from build123d import *

# Parameters (mm, degrees)
SKETCH1_W                = 74.7
SKETCH1_H                = 52.5
BOSS_EXTRUDE1_DEPTH      = 83
SKETCH4_W                = 42.5
SKETCH4_H                = 42.5
CUT_EXTRUDE1_DEPTH       = 24
SKETCH7_R                = 8.6
CUT_EXTRUDE6_DEPTH       = 130
CUT_EXTRUDE16_DEPTH      = 115.708990493
CUT_EXTRUDE16_DEPTH_BACK = 4.99
SKETCH13_W               = 45.5
SKETCH13_H               = 61
SKETCH15_W               = 6.385819608
SKETCH15_H               = 61
CUT_EXTRUDE17_DEPTH      = 1
SKETCH18_W               = 42.5
SKETCH18_H               = 42.5
BOSS_EXTRUDE2_DEPTH      = 31
SKETCH19_W               = 52.25
SKETCH19_H               = 52.5
BOSS_EXTRUDE3_DEPTH      = 50
SKETCH20_W               = 42.5
SKETCH20_H               = 42.5
CUT_EXTRUDE19_DEPTH      = 23.5
SKETCH21_W               = 52.5
SKETCH21_H               = 5
BOSS_EXTRUDE4_DEPTH      = 30
FILLET1_R                = 5
SKETCH22_R               = 15
CUT_EXTRUDE20_DEPTH      = 120
CUT_EXTRUDE21_DEPTH      = 3
SKETCH24_R               = 20
SKETCH24_R_2             = 15
BOSS_EXTRUDE5_DEPTH      = 82
CUT_EXTRUDE22_START      = -82
CUT_EXTRUDE22_DEPTH      = 82


with BuildPart() as part:
    # Sketch1 → Boss-Extrude1 (new body)
    with BuildSketch(Plane(origin=(0, 0, 0), x_dir=(1, 0, 0), z_dir=(0, 1, 0))):
        Rectangle(SKETCH1_W, SKETCH1_H)
    extrude(amount=BOSS_EXTRUDE1_DEPTH)

    # Sketch4 → Cut-Extrude1 (cut)
    with BuildSketch(Plane.XZ):
        with Locations((11.1, 0)):
            Rectangle(SKETCH4_W, SKETCH4_H)
    extrude(amount=-CUT_EXTRUDE1_DEPTH, mode=Mode.SUBTRACT)

    # Sketch7 → Cut-Extrude6 (cut)
    with BuildSketch(Plane.XZ):
        with Locations(Location((-23.75, 0, 0), (0, 0, 270))):
            Circle(SKETCH7_R)
    extrude(amount=-CUT_EXTRUDE6_DEPTH, mode=Mode.SUBTRACT)

    # Sketch13 → Cut-Extrude16 (cut, two sides: drawn at the far end of the back side and taken through both)
    with BuildSketch(Plane.ZY.offset(37.35).offset(-CUT_EXTRUDE16_DEPTH_BACK)):
        with Locations((0, 41.5)):
            Rectangle(SKETCH13_W, SKETCH13_H)
    extrude(amount=CUT_EXTRUDE16_DEPTH + CUT_EXTRUDE16_DEPTH_BACK, mode=Mode.SUBTRACT)

    # Sketch15 → Cut-Extrude17 (cut)
    with BuildSketch(Plane.ZY.offset(32.36)):
        with Locations((0, 41.5)):
            Rectangle(SKETCH15_W, SKETCH15_H)
    extrude(amount=-CUT_EXTRUDE17_DEPTH, mode=Mode.SUBTRACT)

    # Sketch18 → Boss-Extrude2 (add)
    with BuildSketch(Plane.XZ):
        with Locations((11.1, 0)):
            Rectangle(SKETCH18_W, SKETCH18_H)
    extrude(amount=-BOSS_EXTRUDE2_DEPTH)

    # Sketch19 → Boss-Extrude3 (add)
    with BuildSketch(Plane.XZ):
        with Locations((11.225, 0)):
            Rectangle(SKETCH19_W, SKETCH19_H)
    extrude(amount=BOSS_EXTRUDE3_DEPTH)

    # Sketch20 → Cut-Extrude19 (cut)
    with BuildSketch(Plane.XZ.offset(50)):
        with Locations((11.1, 0)):
            Rectangle(SKETCH20_W, SKETCH20_H)
    extrude(amount=-CUT_EXTRUDE19_DEPTH, mode=Mode.SUBTRACT)

    # Sketch21 → Boss-Extrude4 (add)
    with BuildSketch(Plane(origin=(37.35, 0, 0), x_dir=(0, 0, -1), z_dir=(1, 0, 0))):
        with Locations((0, -47.5)):
            Rectangle(SKETCH21_W, SKETCH21_H)
    extrude(amount=BOSS_EXTRUDE4_DEPTH)

    # Fillet1
    fillet1_edges = [part.edges().sort_by_distance(p)[0] for p in [
        (37.35, -45, 0),
    ]]
    fillet(fillet1_edges, radius=FILLET1_R)

    # Sketch22 → Cut-Extrude20 (cut)
    with BuildSketch(Plane.XZ.offset(26.5)):
        with Locations(Location((11.1, 0, 0), (0, 0, 270))):
            Circle(SKETCH22_R)
    extrude(amount=-CUT_EXTRUDE20_DEPTH, mode=Mode.SUBTRACT)

    # Sketch23 → Cut-Extrude21 (cut)
    with BuildSketch(Plane(origin=(0, 83, 0), x_dir=(1, 0, 0), z_dir=(0, 1, 0))):
        Polygon((-16.75, 16), (-12.788538026, -0.140014893), (-16.75, -16), (-30.75, -16), (-34.596459266, 0.235543482), (-30.75, 16), align=None)
    extrude(amount=-CUT_EXTRUDE21_DEPTH, mode=Mode.SUBTRACT)

    # Sketch24 → Boss-Extrude5 (add)
    with BuildSketch(Plane(origin=(0, 83, 0), x_dir=(1, 0, 0), z_dir=(0, 1, 0))):
        with Locations(Location((11.1, 0, 0), (0, 0, 270))):
            Circle(SKETCH24_R)
        with Locations(Location((11.1, 0, 0), (0, 0, 90))):
            Circle(SKETCH24_R_2, mode=Mode.SUBTRACT)
    extrude(amount=BOSS_EXTRUDE5_DEPTH)

    # Sketch27 → Cut-Extrude22 (cut)
    with BuildSketch(Plane(origin=(0, 165, 0), x_dir=(1, 0, 0), z_dir=(0, 1, 0)).offset(CUT_EXTRUDE22_START)):
        with BuildLine():
            Line((-5.423226258, 11.268673126), (1.199646169, 11.268673126))
            ThreePointArc((1.199646169, 11.268673126), (-3.9, 0), (1.199646169, -11.268673126))
            Line((1.199646169, -11.268673126), (-5.423226258, -11.268673126))
            ThreePointArc((-5.423226258, -11.268673126), (-8.9, 0), (-5.423226258, 11.268673126))
        make_face()
    extrude(amount=CUT_EXTRUDE22_DEPTH, mode=Mode.SUBTRACT)


solid = part.part
Can you work these out from the model? Positions are in its coordinate system, mm. A direction names the side the tool comes from. Round coordinates to 2 decimals unless told otherwise and drop trailing zeros. Write each loop counter-clockwise with the first axis right and the second up, starting at its lowest first coordinate (ties: lowest second). Pieces come first, ordered by that corner, then holes. Notation, with made-up numbers: M 72,-8 L 93,-8 A32 ccw 93,18 Z; hole C -32,-36 d8. An arc over 180 degrees is marked long. Use a Markdown table: item, result.
Item 1: Which directions (+Z, -Z, +X, -X, +Y, -Y) give clear straight access to the entire face, cutting with the end or side of a thin tool? Please do faces 4 (the face through (55, -45, 0)), 5 (the face through (-18.7, 80, -7.3)), 6 (the face through (-2, 123, 11.269)).
Found:
| item | result |
|---|---|
| face 4 | +Z, -Z, +X, +Y |
| face 5 | +Y |
| face 6 | -X, +Y |
Item 2: If I drill on line 1 along X through (y, z) = (16, 0); line 2 along Z through (x, y) = (7.5, -31); line 3 along Y through (x, z) = (0, -21), over which ranges is the centre line in solid material (lowest first)? Write a range as [from, to].
Found:
| item | result |
|---|---|
| line 1 | x = [-15.15, -3.9], [26.1, 37.35] |
| line 2 | z = [-26.25, -21.25], [21.25, 26.25] |
| line 3 | y = [-26.5, 83] |
Item 3: I want a section at C-C (x = -23.75). List the corners of the cut face in (y, z) for me, and give its area (3 significant figures).
Found:
| item | result |
|---|---|
| outline | M 0,-26.25 L 83,-26.25 L 83,-16 L 80,-16 L 80,-8.6 L 0,-8.6 Z; M 0,8.6 L 80,8.6 L 80,16 L 83,16 L 83,26.25 L 0,26.25 Z |
| area | 2,890 mm2 |
Item 4: We'd pull the mould along Z, two halves only. Please class faces 1 (the face through (67.35, -47, 0)), 2 (the face through (-35, 11, 0)), 3 (the face through (-32.7, 81.5, -8)): released by +Z, released by -Z, zero draft, split by the parting line, or undercut.
Found:
| item | result |
|---|---|
| face 1 | zero draft |
| face 2 | undercut |
| face 3 | undercut |
Item 5: I want a section at A-A (x = 11.1). List the corners of the cut face in (y, z) for me, and give its area (3 significant figures).
Found:
| item | result |
|---|---|
| outline | M -50,-26.25 L 83,-26.25 L 83,-20 L 165,-20 L 165,-15 L -26.5,-15 L -26.5,-21.25 L -50,-21.25 Z; M -50,21.25 L -26.5,21.25 L -26.5,15 L 165,15 L 165,20 L 83,20 L 83,26.25 L -50,26.25 Z |
| area | 3,520 mm2 |
Item 6: I want a section at B-B (y = -31.5). List the corners of the cut face in (x, z) for me, and give its area (3 significant figures).
Found:
| item | result |
|---|---|
| outline | M -14.9,-26.25 L 37.35,-26.25 L 37.35,26.25 L -14.9,26.25 Z; hole M -10.15,-21.25 L 32.35,-21.25 L 32.35,21.25 L -10.15,21.25 Z |
| area | 937 mm2 |
Item 7: For pin 1 Ø1.7 at (x, z) = (-35, 7.5) entering from +Y; pin 2 Ø21.5 at (y, z) = (39, -9.5) entering from -X; pin 3 Ø7.5 at (x, y) = (-1, 111.5) entering from -Z, each with a flat end and sliding along its axis, tell me the tip position at first contact or that it passes through.
Found:
| item | result |
|---|---|
| pin 1 | stops at y = 83 |
| pin 2 | stops at x = -32.36 |
| pin 3 | stops at z = -18.17 |
Item 8: I want a section at D-D (y = 59). List the corners of the cut face in (x, z) for me.
Found:
| item | result |
|---|---|
| outline | M -37.35,-26.25 L 37.35,-26.25 L 37.35,26.25 L -37.35,26.25 L -37.35,22.75 L -32.36,22.75 L -32.36,3.19 L -31.74,3.19 A8.6 cw long -31.74,-3.19 L -32.36,-3.19 L -32.36,-22.75 L -37.35,-22.75 Z; hole C 11.1,0 d30 |
